Geometry check sheet. Reference: drawing and pictorial views, mm from the part's lowest x, y, z. Give positions to 0.01 mm unless a question says otherwise; leave off trailing zeros. Order: outer loops, then holes, each group sorted by start corner. A loop starts at its lowest first (then second) coordinate and runs counter-clockwise, first axis right, second up.
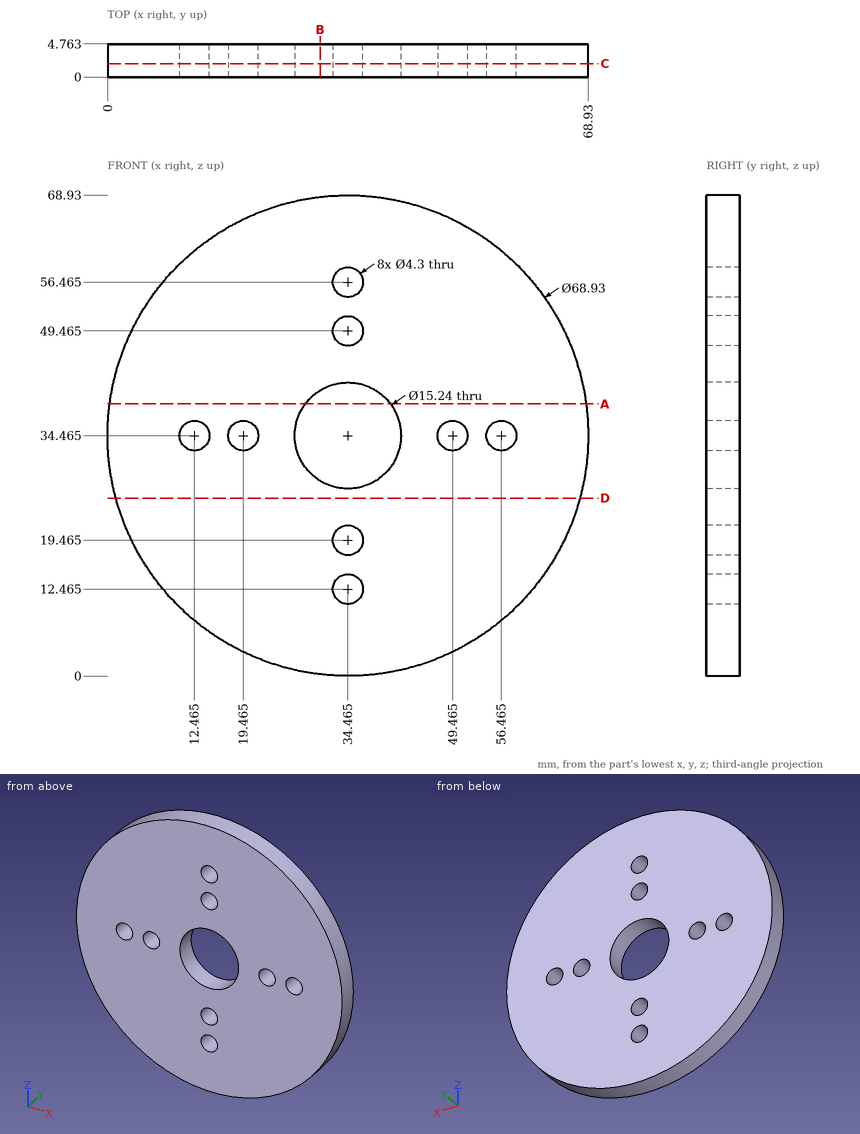
(1) Material ranges on L1, parallel to X at y = 1.45, z = 14 (1 decimal); L2, parallel to Z at x = 30.5, y = 1.4; L3, parallel to X at y = 4.2, z = 48, recorded low to high.
Response values:
L1: x = 6.7 to 33, 36 to 62.2
L2: z = 0.23 to 27.96, 40.97 to 68.7
L3: x = 2.77 to 32.89, 36.04 to 66.16
(2) Cross-section at B-B on x = 30.5. Enter the section's corners in (y, z), then the cut area to 3 significant figures.
Response values:
outline: (0, 0.23) - (4.76, 0.23) - (4.76, 27.96) - (0, 27.96) - close; (0, 40.97) - (4.76, 40.97) - (4.76, 68.7) - (0, 68.7) - close
area: 264 mm2
(3) Gauge pin test, flat ends, axial feed: pin 1 Ø2 at (y, z) = (2.5, 26) entering from -X; pin 2 Ø2 at (x, y) = (44.5, 1.5) entering from +Z (1 decimal). Record the tip position at first contact, or that the pin passes through.
Response values:
pin 1: stops at x = 0.82
pin 2: stops at z = 67.7
(4) Cross-section at D-D on z = 25.5. Enter the section's corners in (x, y).
Response values:
outline: (1.19, 0) - (67.74, 0) - (67.74, 4.76) - (1.19, 4.76) - close
(5) Cross-section at C-C on y = 1.95. Count the separate pieces of the cut face and the enclosed holes in it, then the cut area to 3 significant figures.
Response values:
separate pieces: 1
enclosed holes: 9
area: 3,430 mm2
(6) Cross-section at A-A on z = 39. Enter the section's corners in (x, y), then the cut area to 3 significant figures.
Response values:
outline: (0.3, 0) - (28.34, 0) - (28.34, 4.76) - (0.3, 4.76) - close; (40.59, 0) - (68.63, 0) - (68.63, 4.76) - (40.59, 4.76) - close
area: 267 mm2
